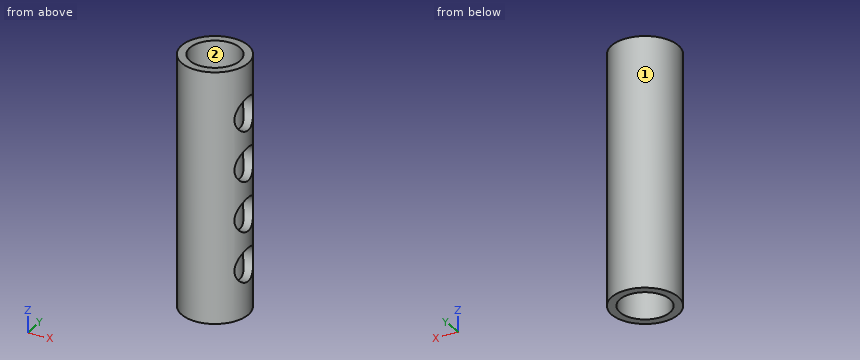
```python
from build123d import *

# Parameters (mm, degrees)
SKETCH1_R           = 4
BOSS_EXTRUDE1_DEPTH = 30
SKETCH2_R           = 3
CUT_EXTRUDE1_DEPTH  = 31
CUT_EXTRUDE2_START  = 5
SKETCH3_R           = 2
CUT_EXTRUDE2_DEPTH  = 4


with BuildPart() as part:
    # Sketch1 → Boss-Extrude1 (new body)
    with BuildSketch(Plane.XY):
        Circle(SKETCH1_R)
    extrude(amount=BOSS_EXTRUDE1_DEPTH)

    # Sketch2 → Cut-Extrude1 (cut, through all)
    with BuildSketch(Plane.XY.offset(30)):
        Circle(SKETCH2_R)
    extrude(amount=-CUT_EXTRUDE1_DEPTH, mode=Mode.SUBTRACT)

    # Sketch3 → Cut-Extrude2 (cut)
    with BuildSketch(Plane(origin=(0, 0, 0), x_dir=(0, 0, -1), z_dir=(1, 0, 0)).offset(CUT_EXTRUDE2_START)):
        with Locations((-6, 0)):
            Circle(SKETCH3_R)
        with Locations((-12, 0)):
            Circle(SKETCH3_R)
        with Locations((-18, 0)):
            Circle(SKETCH3_R)
        with Locations((-24, 0)):
            Circle(SKETCH3_R)
    extrude(amount=-CUT_EXTRUDE2_DEPTH, mode=Mode.SUBTRACT)


solid = part.part
```
Read the model definition and answer for the solid it produces. Units are mm, in the model's axes. Face numbers are marked on the shaded views. Give positions to 0.01 mm unless a question says otherwise; leave off trailing zeros. Write each loop counter-clockwise with the first axis right and the second up, starting at its lowest first coordinate (ties: lowest second). Pieces come first, ordered by that corner, then holes. Notation, with made-up numbers: (76.25, 13.25) -> (112.25, 13.25) arc R23 cw to (112.25, 26.25) -> close; hole circle Ø10 at (61, -26.5). An arc over 180 degrees is marked (long way). Answer in a Markdown table with one row per item.
1) Section C-C on z = 27.5 is taken. Give the vertices of the cut face in (x, y).
Results list:
| item | result |
|---|---|
| outline | circle Ø8 at (0, 0); hole circle Ø6 at (0, 0) |
2) Section D-D on z = 12 is taken. Give the vertices of the cut face in (x, y).
Results list:
| item | result |
|---|---|
| outline | (2.24, -2) arc R3 cw (long way) to (2.24, 2) -> (3.46, 2) arc R4 ccw (long way) to (3.46, -2) -> close |
3) Determine the mould class of the marked faces 1 and 2 for opening direction X: released by +X, released by -X, zero draft, split by the parting line, or undercut.
Results list:
| item | result |
|---|---|
| face 1 | split by the parting line |
| face 2 | undercut |
4) Straight lines are drawn through the part: line 1 (Z direction, x = 3.55, y = 0); line 2 (Y direction, x = 0, z = 21); line 3 (Z direction, x = 2.75, y = 1.5). For each, find the intervals that lie inside material, in ascending order. Write a range as [from, to].
Results list:
| item | result |
|---|---|
| line 1 | [0, 4], [8, 10], [14, 16], [20, 22], [26, 30] |
| line 2 | [-4, -3], [3, 4] |
| line 3 | [0, 4.68], [7.32, 10.68], [13.32, 16.68], [19.32, 22.68], [25.32, 30] |
5) Section B-B on x = 0.5 is taken. Give the vertices of the cut face in (y, z).
Results list:
| item | result |
|---|---|
| outline | (-3.97, 0) -> (-2.96, 0) -> (-2.96, 30) -> (-3.97, 30) -> close; (2.96, 0) -> (3.97, 0) -> (3.97, 30) -> (2.96, 30) -> close |
6) Each of these flat-tipped pins is pushed along its axis until it touches: pin 1 Ø1.5 at (y, z) = (-3, 19) entering from -X; pin 2 Ø2.5 at (y, z) = (0, 6) entering from +X. Where does it stop, or does it pass through?
Results list:
| item | result |
|---|---|
| pin 1 | x = -3.31 |
| pin 2 | x = -2.73 |
7) Section A-A on y = 0 is taken. Give the vertices of the cut face in (x, z).
Results list:
| item | result |
|---|---|
| outline | (-4, 0) -> (-3, 0) -> (-3, 30) -> (-4, 30) -> close; (3, 0) -> (4, 0) -> (4, 4) -> (3, 4) -> close; (3, 8) -> (4, 8) -> (4, 10) -> (3, 10) -> close; (3, 14) -> (4, 14) -> (4, 16) -> (3, 16) -> close; (3, 20) -> (4, 20) -> (4, 22) -> (3, 22) -> close; (3, 26) -> (4, 26) -> (4, 30) -> (3, 30) -> close |
